from build123d import *

# Parameters (mm, degrees)
SKETCH2_R                        = 17.4625
SKETCH2_R_2                      = 15.875
BOSS_EXTRUDE1_DEPTH              = 266.7
F_6_CLEARANCE_HOLE1_D            = 3.7973
F_1_4_0_25_DIAMETER_HOLE1_REACH  = 36.925
F_1_4_0_25_DIAMETER_HOLE1_BORE_R = 3.175


with BuildPart() as part:
    # Sketch2 → Boss-Extrude1 (new body)
    with BuildSketch(Plane.XY):
        Circle(SKETCH2_R)
        Circle(SKETCH2_R_2, mode=Mode.SUBTRACT)
    extrude(amount=BOSS_EXTRUDE1_DEPTH)

    # #6 Clearance Hole1 (through all)
    with Locations(Plane(origin=(17.4625, 0, 19.05), x_dir=(0, 1, 0), z_dir=(1, 0, 0))):
        with Locations((0, 0)):
            Hole(F_6_CLEARANCE_HOLE1_D / 2)

    # 1/4 (0.25) Diameter Hole1 bore (on position points) → 1/4 (0.25) Diameter Hole1 (cut, up to next)
    with BuildSketch(Plane(origin=(17.4625, 0, 38.1), x_dir=(0, 1, 0), z_dir=(1, 0, 0)), mode=Mode.PRIVATE) as f_1_4_0_25_diameter_hole1_sk1:
        Circle(F_1_4_0_25_DIAMETER_HOLE1_BORE_R)
    f_1_4_0_25_diameter_hole1_tool1 = extrude(f_1_4_0_25_diameter_hole1_sk1.sketch, amount=-F_1_4_0_25_DIAMETER_HOLE1_REACH, mode=Mode.PRIVATE) & part.part
    add(f_1_4_0_25_diameter_hole1_tool1.solids().sort_by_distance((17.4625, 0, 38.1))[0], mode=Mode.SUBTRACT)


solid = part.part
Check sheet for the modelled part. Datum: model origin and axes. Units: mm. A direction names the side the tool comes from. Give positions to 0.01 mm unless a question says otherwise; leave off trailing zeros. Order: outer loops, then holes, each group sorted by start corner. A loop starts at its lowest first (then second) coordinate and runs counter-clockwise, first axis right, second up. Notation, with made-up numbers: (17.25, 15.25) - (38.25, 15.25) arc R24 ccw to (38.25, 54.25) - close; hole circle Ø3 at (48.25, 0.5). An arc over 180 degrees is marked (long way). Answer as CSV lines item,"result".
1. Section check B-B (y = -9). Record the boundary of the cut face in (x, z), then the cut area to 3 significant figures.
Result sheet:
outline,"(-14.96, 0) - (-13.08, 0) - (-13.08, 266.7) - (-14.96, 266.7) - close; (13.08, 0) - (14.96, 0) - (14.96, 266.7) - (13.08, 266.7) - close"
area,"1,010 mm²"
2. Section check A-A (x = 0). Record the boundary of the cut face in (y, z) (1 decimal).
Result sheet:
outline,"(-17.5, 0) - (-15.9, 0) - (-15.9, 266.7) - (-17.5, 266.7) - close; (15.9, 0) - (17.5, 0) - (17.5, 266.7) - (15.9, 266.7) - close"
3. Tool access check on faces 1 (the face through (8, -14, 266.7)), 2 (the face through (16.52, 2.93, 36.88)). Record the directions out of +Z, -Z, +X, -X, +Y, -Y that give a thin tool (end or side, any length) a straight path to the whole face; none if there is none.
Result sheet:
face 1,"+Z, +X, -X, +Y, -Y"
face 2,"+X"
4. Go/stop test with flat-tipped pins: P1, Ø6, axis at x = 10.5, z = 200, coming from the -Y side; P2, Ø19, axis at x = 0, y = 0, coming from the +Z side; P3, Ø1.5, axis at y = 7, z = 234, coming from the +X side; P4, Ø4, axis at y = 9, z = 230.5, coming from the -X side. Record where each tip stops, or that it passes through.
Result sheet:
P1,"y = -15.77"
P2,"through"
P3,"x = 16.31"
P4,"x = -16"
5. Mould release check, pull along X, two halves, no side actions. Record for faces 3 (the face through (8, -14, 0)), 4 (the face through (-13.858, -10.626, 131.483)), 5 (the face through (-3.441, -15.497, 131.483)): released by +X, released by -X, zero draft, split by the parting line, or undercut.
Result sheet:
face 3,"zero draft"
face 4,"split by the parting line"
face 5,"undercut"
6. Scan lines: probe 1 along Y at (x, z) = (0, 89.5) (1 decimal); probe 2 along Y at (x, z) = (1, 71). Record each from-to range of solid material in increasing order. Write a range as from..to.
Result sheet:
probe 1,"-17.5..-15.9, 15.9..17.5"
probe 2,"-17.43..-15.84, 15.84..17.43"
